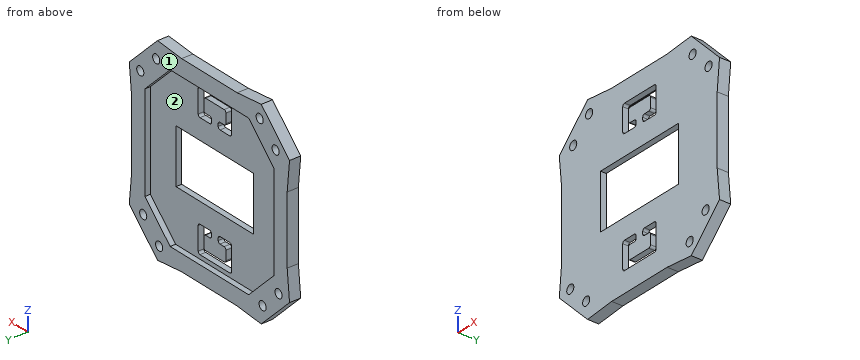
```python
from build123d import *

# Parameters (mm, degrees)
SKETCH1_R           = 1.6
BOSS_EXTRUDE2_DEPTH = 4.1
CUT_EXTRUDE1_DEPTH  = 2
CUT_EXTRUDE4_DEPTH  = 52.043216983
SKETCH9_W           = 35
SKETCH9_H           = 20
CUT_EXTRUDE5_DEPTH  = 10


with BuildPart() as part:
    # Sketch1 → Boss-Extrude2 (new body)
    with BuildSketch(Plane(origin=(0, 0, 0), x_dir=(1, 0, 0), z_dir=(0, 1, 0))):
        Polygon((-12.5, 35), (12.5, 35), (23.334523779, 36.062445841), (36.062445841, 23.334523779), (35, 12.5), (35, -12.5), (36.062445841, -23.334523779), (23.334523779, -36.062445841), (12.5, -35), (-12.5, -35), (-23.334523779, -36.062445841), (-36.062445841, -23.334523779), (-35, -12.5), (-35, 12.5), (-36.062445841, 23.334523779), (-23.334523779, 36.062445841), align=None)
        with Locations(Location((22.627416998, 31.112698372, 0), (0, 0, 270))):
            Circle(SKETCH1_R, mode=Mode.SUBTRACT)
        with Locations(Location((29.79056362, 23.94955175, 0), (0, 0, 270))):
            Circle(SKETCH1_R, mode=Mode.SUBTRACT)
        with Locations(Location((31.112698372, -22.627416998, 0), (0, 0, 270))):
            Circle(SKETCH1_R, mode=Mode.SUBTRACT)
        with Locations(Location((23.94955175, -29.79056362, 0), (0, 0, 270))):
            Circle(SKETCH1_R, mode=Mode.SUBTRACT)
        with Locations(Location((-22.627416998, -31.112698372, 0), (0, 0, 270))):
            Circle(SKETCH1_R, mode=Mode.SUBTRACT)
        with Locations(Location((-29.79056362, -23.94955175, 0), (0, 0, 270))):
            Circle(SKETCH1_R, mode=Mode.SUBTRACT)
        with Locations(Location((-31.112698372, 22.627416998, 0), (0, 0, 270))):
            Circle(SKETCH1_R, mode=Mode.SUBTRACT)
        with Locations(Location((-23.94955175, 29.79056362, 0), (0, 0, 270))):
            Circle(SKETCH1_R, mode=Mode.SUBTRACT)
    extrude(amount=BOSS_EXTRUDE2_DEPTH)

    # Sketch2 → Cut-Extrude1 (cut)
    with BuildSketch(Plane(origin=(0, 4.1, 0), x_dir=(1, 0, 0), z_dir=(0, 1, 0))):
        Polygon((-17.669047558, 29), (17.669047558, 29), (29, 17.669047558), (29, -17.669047558), (17.669047558, -29), (-17.669047558, -29), (-29, -17.669047558), (-29, 17.669047558), align=None)
    extrude(amount=-CUT_EXTRUDE1_DEPTH, mode=Mode.SUBTRACT)

    # Sketch8 → Cut-Extrude4 (cut, through all)
    with BuildSketch(Plane(origin=(0, 2.1, 0), x_dir=(1, 0, 0), z_dir=(0, 1, 0))):
        with BuildLine():
            Line((-1.5, 19.18174342), (-1.5, 18.3))
            ThreePointArc((-1.5, 18.3), (-1.734314575, 17.734314575), (-2.3, 17.5))
            Line((-2.3, 17.5), (-6.7, 17.5))
            ThreePointArc((-6.7, 17.5), (-7.265685425, 17.734314575), (-7.5, 18.3))
            Line((-7.5, 18.3), (-7.5, 26.7))
            ThreePointArc((-7.5, 26.7), (-7.265685425, 27.265685425), (-6.7, 27.5))
            Line((-6.7, 27.5), (6.7, 27.5))
            ThreePointArc((6.7, 27.5), (7.265685425, 27.265685425), (7.5, 26.7))
            Line((7.5, 26.7), (7.5, 18.3))
            ThreePointArc((7.5, 18.3), (7.265685425, 17.734314575), (6.7, 17.5))
            Line((6.7, 17.5), (2.3, 17.5))
            ThreePointArc((2.3, 17.5), (1.734314575, 17.734314575), (1.5, 18.3))
            Line((1.5, 18.3), (1.5, 19.18174342))
            ThreePointArc((1.5, 19.18174342), (1.734314575, 19.747428845), (2.3, 19.98174342))
            Line((2.3, 19.98174342), (4.2, 19.98174342))
            ThreePointArc((4.2, 19.98174342), (4.765685425, 20.216057995), (5, 20.78174342))
            Line((5, 20.78174342), (5, 24.21825658))
            ThreePointArc((5, 24.21825658), (4.765685425, 24.783942005), (4.2, 25.01825658))
            Line((4.2, 25.01825658), (-4.2, 25.01825658))
            ThreePointArc((-4.2, 25.01825658), (-4.765685425, 24.783942005), (-5, 24.21825658))
            Line((-5, 24.21825658), (-5, 20.78174342))
            ThreePointArc((-5, 20.78174342), (-4.765685425, 20.216057995), (-4.2, 19.98174342))
            Line((-4.2, 19.98174342), (-2.3, 19.98174342))
            ThreePointArc((-2.3, 19.98174342), (-1.734314575, 19.747428845), (-1.5, 19.18174342))
        make_face()
        with BuildLine():
            Line((2.3, -17.5), (6.7, -17.5))
            ThreePointArc((6.7, -17.5), (7.265685425, -17.734314575), (7.5, -18.3))
            Line((7.5, -18.3), (7.5, -26.7))
            ThreePointArc((7.5, -26.7), (7.265685425, -27.265685425), (6.7, -27.5))
            Line((6.7, -27.5), (-6.7, -27.5))
            ThreePointArc((-6.7, -27.5), (-7.265685425, -27.265685425), (-7.5, -26.7))
            Line((-7.5, -26.7), (-7.5, -18.3))
            ThreePointArc((-7.5, -18.3), (-7.265685425, -17.734314575), (-6.7, -17.5))
            Line((-6.7, -17.5), (-2.3, -17.5))
            ThreePointArc((-2.3, -17.5), (-1.734314575, -17.734314575), (-1.5, -18.3))
            Line((-1.5, -18.3), (-1.5, -19.18174342))
            ThreePointArc((-1.5, -19.18174342), (-1.734314575, -19.747428845), (-2.3, -19.98174342))
            Line((-2.3, -19.98174342), (-4.2, -19.98174342))
            ThreePointArc((-4.2, -19.98174342), (-4.765685425, -20.216057995), (-5, -20.78174342))
            Line((-5, -20.78174342), (-5, -24.21825658))
            ThreePointArc((-5, -24.21825658), (-4.765685425, -24.783942005), (-4.2, -25.01825658))
            Line((-4.2, -25.01825658), (4.2, -25.01825658))
            ThreePointArc((4.2, -25.01825658), (4.765685425, -24.783942005), (5, -24.21825658))
            Line((5, -24.21825658), (5, -20.78174342))
            ThreePointArc((5, -20.78174342), (4.765685425, -20.216057995), (4.2, -19.98174342))
            Line((4.2, -19.98174342), (2.3, -19.98174342))
            ThreePointArc((2.3, -19.98174342), (1.734314575, -19.747428845), (1.5, -19.18174342))
            Line((1.5, -19.18174342), (1.5, -18.3))
            ThreePointArc((1.5, -18.3), (1.734314575, -17.734314575), (2.3, -17.5))
        make_face()
    extrude(amount=-CUT_EXTRUDE4_DEPTH, mode=Mode.SUBTRACT)

    # Sketch9 → Cut-Extrude5 (cut)
    with BuildSketch(Plane(origin=(0, 2.1, 0), x_dir=(1, 0, 0), z_dir=(0, 1, 0))):
        Rectangle(SKETCH9_W, SKETCH9_H)
    extrude(amount=-CUT_EXTRUDE5_DEPTH, mode=Mode.SUBTRACT)


solid = part.part
```
The model under review builds one solid part; all positions refer to its coordinate system, in mm. Face numbers are marked on the shaded views. Round coordinates to 2 decimals unless told otherwise and drop trailing zeros. Order: outer loops, then holes, each group sorted by start corner. A loop starts at its lowest first (then second) coordinate and runs counter-clockwise, first axis right, second up. Notation, with made-up numbers: (-12, 18) -> (-7, 18) arc R8 cw to (-7, 27) -> close; hole circle Ø7 at (81.25, 52). An arc over 180 degrees is marked (long way). One line per item, written item: value. Start each with the question number.
Q1. Take a section at B-B (y = 2.75). Count the separate pieces of the cut face and the enclosed holes in it, and give its area (3 significant figures).
Q2. Take a section at C-C (x = 20). Write out the cut boundary in (y, z), and give its area (3 significant figures).
Q3. Take a section at A-A (x = 9.5). Write out the cut boundary in (y, z), and give its area (3 significant figures).
Q4. Clearance check with flat-ended pins moving along their axes: pin 1 Ø2 at (x, z) = (24.5, 8) entering from +Y; pin 2 Ø2 at (x, y) = (-14.5, 1) entering from -Z; pin 3 Ø2.5 at (x, z) = (-23.95, -29.79) entering from -Y; pin 4 Ø1.6 at (x, y) = (8.5, 3.5) entering from +Z. State where each tip first meets the part, or that it passes through.
Q5. Wall thickness on line 1 (X direction, y = 2.9, z = -6.5); line 2 (X direction, y = 1.4, z = -9); line 3 (Z direction, x = 23, y = 3.3): over which ranges is each line inside the solid? List them lowest first.
Q6. Mouldability with a two-part tool opening along X and no side actions: class the marked faces 1 and 2 as released by +X, released by -X, zero draft, split by the parting line, or undercut.
Q7. Take a section at D-D (z = 14.5). Write out the cut boundary in (x, y).
Reported:
1. separate pieces: 1
1. enclosed holes: 9
1. area: 1,550 mm2
2. outline: (0, -35.74) -> (4.1, -35.74) -> (4.1, -26.67) -> (2.1, -26.67) -> (2.1, 26.67) -> (4.1, 26.67) -> (4.1, 35.74) -> (0, 35.74) -> close
2. area: 186 mm2
3. outline: (0, -35) -> (4.1, -35) -> (4.1, -29) -> (2.1, -29) -> (2.1, -10) -> (0, -10) -> close; (0, 10) -> (2.1, 10) -> (2.1, 29) -> (4.1, 29) -> (4.1, 35) -> (0, 35) -> close
3. area: 129 mm2
4. pin 1: stops at y = 2.1
4. pin 2: stops at z = -35.29
4. pin 3: passes through
4. pin 4: stops at z = 35
5. line 1: x = -35 to -29, 29 to 35
5. line 2: x = -35 to -17.5, 17.5 to 35
5. line 3: z = -36.03 to -32.67, -29.56 to -23.67, 23.67 to 28.5, 31.08 to 36.03
6. face 1: zero draft
6. face 2: undercut
7. outline: (-35.2, 0) -> (35.2, 0) -> (35.2, 4.1) -> (29, 4.1) -> (29, 2.1) -> (-29, 2.1) -> (-29, 4.1) -> (-35.2, 4.1) -> close
